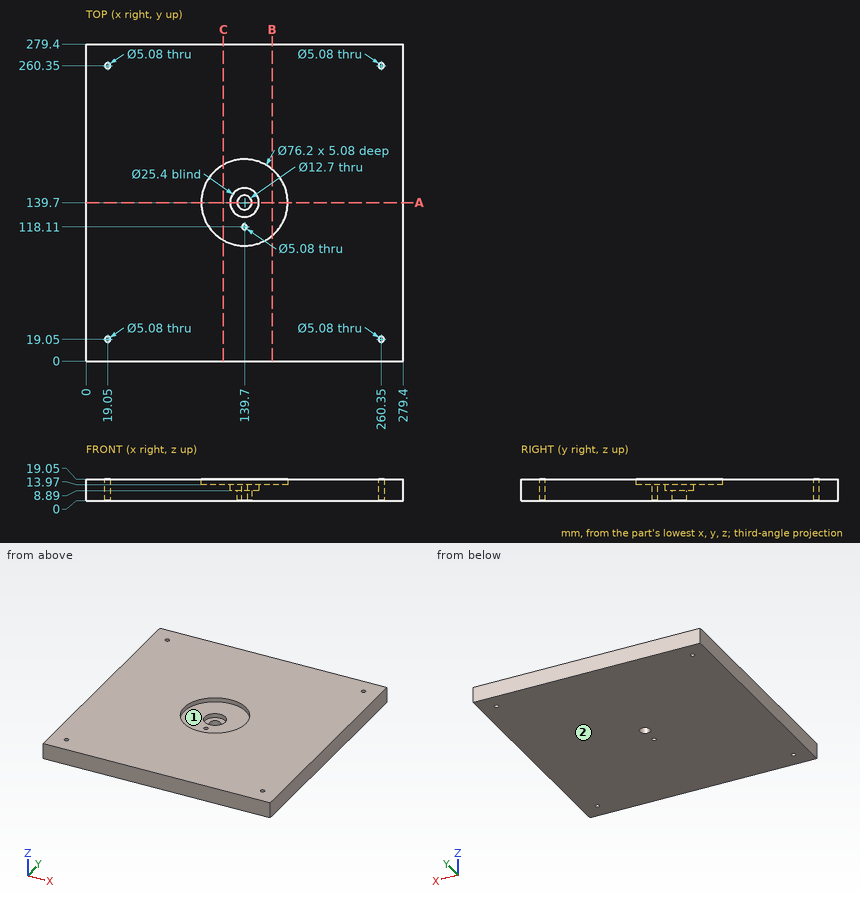
Input: dimensioned drawing with shaded views. Units: mm. Origin: part minimum x, y, z. Round coordinates to 2 decimals unless told otherwise and drop trailing zeros. Order: outer loops, then holes, each group sorted by start corner. A loop starts at its lowest first (then second) coordinate and runs counter-clockwise, first axis right, second up. Notation, with made-up numbers: (70.5, 16) -> (126.5, 16) arc R11 ccw to (126.5, 27) -> close; hole circle Ø9 at (-11, -35). An arc over 180 degrees is marked (long way). One line per item, written item: value. Start each with the question number.
Q1. Material intervals for probe 1 along Y at (x, z) = (139.7, 8); probe 2 along X at (y, z) = (260.35, 13.25); probe 3 along Y at (x, z) = (139.7, 12.6), sorted ascending.
Q2. Pin query (flat end, axial travel): pin 1 (16.5 mm diameter, centred on x = 139.7, y = 139.7, fed in from +Z); pin 2 (5 mm diameter, centred on x = 182.5, z = 12, fed in from -Y); pin 3 (4 mm diameter, centred on x = 139.7, y = 118.11, fed in from -Z). Return the tip coordinate at first contact, or that it passes through.
Q3. Section query C-C (x = 121). Return the cut outline in (y, z), plus the area to 3 significant figures.
Q4. Draft query along X for the marked faces 1 and 2. Return one class per face: pulls with the +X half, pulls with the -X half, needs draft (parallel to the pull), parting line crosses it, or undercut.
Q5. Section query B-B (x = 164). Return the cut outline in (y, z).
Q6. Section query A-A (y = 139.7). Return the cut outline in (x, z).
Findings below:
1. probe 1: 0 to 115.57, 120.65 to 133.35, 146.05 to 279.4
1. probe 2: 0 to 16.51, 21.59 to 257.81, 262.89 to 279.4
1. probe 3: 0 to 115.57, 120.65 to 127, 152.4 to 279.4
2. pin 1: z = 8.89
2. pin 2: y = 0
2. pin 3: through
3. outline: (0, 0) -> (279.4, 0) -> (279.4, 19.05) -> (172.9, 19.05) -> (172.9, 13.97) -> (106.5, 13.97) -> (106.5, 19.05) -> (0, 19.05) -> close
3. area: 4,990 mm²
4. face 1: undercut
4. face 2: needs draft
5. outline: (0, 0) -> (279.4, 0) -> (279.4, 19.05) -> (169.04, 19.05) -> (169.04, 13.97) -> (110.36, 13.97) -> (110.36, 19.05) -> (0, 19.05) -> close
6. outline: (0, 0) -> (133.35, 0) -> (133.35, 8.89) -> (127, 8.89) -> (127, 13.97) -> (101.6, 13.97) -> (101.6, 19.05) -> (0, 19.05) -> close; (146.05, 0) -> (279.4, 0) -> (279.4, 19.05) -> (177.8, 19.05) -> (177.8, 13.97) -> (152.4, 13.97) -> (152.4, 8.89) -> (146.05, 8.89) -> close
